from build123d import *

# Parameters (mm, degrees)
F0_W          = 15
F0_H          = 40
F0_W_2        = 20
F0_H_2        = 15
F1_DEPTH      = 30
F2_R          = 25
F2_R_2        = 15
F3_DEPTH      = 20
F3_DEPTH_BACK = 20
F4_DEPTH      = 60
F4_DEPTH_BACK = 60
F5_R          = 12
F7_DEPTH      = 30


with BuildPart() as f1:
    # F0 (on Top) → F1 (new body)
    with BuildSketch(Plane.XY):
        with Locations((-42.5, 20)):
            Rectangle(F0_W, F0_H)
        with BuildLine():
            ThreePointArc((-35, 40), (-29.638939348, 56.069469674), (-20, 70))
            Line((-20, 70), (-20, 85))
            ThreePointArc((-20, 85), (-39.1974084264, 65.2982722843), (-50, 40))
            Line((-50, 40), (-35, 40))
        make_face()
        with Locations((-10, 77.5)):
            Rectangle(F0_W_2, F0_H_2)
        with Locations((10, 77.5)):
            Rectangle(F0_W_2, F0_H_2)
        with BuildLine():
            ThreePointArc((20, 70), (29.638939348, 56.069469674), (35, 40))
            Line((35, 40), (50, 40))
            ThreePointArc((50, 40), (39.1974084264, 65.2982722843), (20, 85))
            Line((20, 85), (20, 70))
        make_face()
        with Locations((42.5, 20)):
            Rectangle(F0_W, F0_H)
    extrude(amount=F1_DEPTH)



with BuildPart() as f3:
    # F2 (on Right) → F3 (new body, two sides)
    with BuildSketch(Plane.YZ) as f3_sk:
        with Locations((0, 15)):
            Circle(F2_R)
        with Locations((0, 15)):
            Circle(F2_R_2, mode=Mode.SUBTRACT)
    extrude(amount=F3_DEPTH)
    extrude(f3_sk.sketch, amount=-F3_DEPTH_BACK)


with BuildPart() as f4:
    # F2 (on Right) → F4 (new body, two sides)
    with BuildSketch(Plane.YZ) as f4_sk:
        with Locations((0, 15)):
            Circle(F2_R_2)
    extrude(amount=F4_DEPTH)
    extrude(f4_sk.sketch, amount=-F4_DEPTH_BACK)

    # F5
    f5_edges = [f4.edges().sort_by_distance(p)[0] for p in [
        (-60, -15, 15),
        (60, -15, 15),
    ]]
    fillet(f5_edges, radius=F5_R)


with BuildPart() as f1_1:
    add(f1.part)

    add(f3.part)  # F7 merges F3

    add(f4.part)  # F7 merges F4
    # F6 (on face) → F7 (join)
    with BuildSketch(Plane(origin=(-50, 0, 0), x_dir=(0, -1, 0), z_dir=(-1, 0, 0))):
        with BuildLine():
            ThreePointArc((0, 0), (-15, 15), (0, 30))
            Line((0, 30), (-5.5677643628, 30))
            ThreePointArc((-5.5677643628, 30), (-16, 15), (-5.5677643628, 0))
            Line((-5.5677643628, 0), (0, 0))
        make_face()
        with BuildLine():
            Line((-5.5677643628, 30), (0, 30))
            ThreePointArc((0, 30), (10.6066017178, 25.6066017178), (15, 15))
            ThreePointArc((15, 15), (10.6066017178, 4.3933982822), (0, 0))
            Line((0, 0), (-5.5677643628, 0))
            ThreePointArc((-5.5677643628, 0), (9.1355287257, 1.8644712743), (16, 15))
            ThreePointArc((16, 15), (9.1355287257, 28.1355287257), (-5.5677643628, 30))
        make_face()
    extrude(amount=-F7_DEPTH)

    # F8: F1 across plane


with BuildPart() as f1_2:
    add(f1_1.part)
    add(f1_1.part.mirror(Plane.YZ))


solid = f1_2.part
Design review of the part built by this model. Coordinates are the model's own, in mm. A direction names the side the tool comes from. Round coordinates to 2 decimals unless told otherwise and drop trailing zeros. Loops run counter-clockwise (first coordinate to the right, second up) from the corner with the lowest first, then second, coordinate; pieces in that order, holes last. Notation, with made-up numbers: (5, 25.25) -> (62, 25.25) arc R26 cw to (62, 45.25) -> close; hole circle Ø11 at (3, 49.25). An arc over 180 degrees is marked (long way). Use one line per item in the form item = value. Start each with the question number.
Q1. We need section B-B on x = 8.5. Give the boundary of the cut face in (y, z).
Q2. We need section A-A on y = 66.5. Give the boundary of the cut face in (x, z).
Q3. For pin 1 Ø1.5 at (y, z) = (63, 28) entering from +X; pin 2 Ø8 at (y, z) = (21.5, 16.5) entering from -X; pin 3 Ø24 at (y, z) = (28, 18.5) entering from +X, all flat-tipped, find the tip position at first contact; note any pin that passes through.
Q4. We need section D-D on z = -6. Give the boundary of the cut face in (x, y), then the cut area to 3 significant figures.
Q5. Wall thickness on line 1 along X through (y, z) = (40, 5); line 2 along X through (y, z) = (18, 21); line 3 along Z through (x, y) = (-12, 79): over which ranges is each line inside the solid? List them lowest first. Write a range as [from, to].
Q6. Draft analysis for pull direction X (two halves, no side actions). For faces 4 (the face through (-20, -0.3, -1.3)), 5 (the face through (50, 25, 15)), 6 (the face through (-38.98, 65.62, 14.79)), state which applies: +X half, -X half, draft (parallel to the pull), parting line (faces both ways), or undercut.
Q7. Machinability: for faces 1 (the face through (-29.745, 55.856, 14.79)), 2 (the face through (39.41, 64.98, 14.79)), 3 (the face through (20, -0.3, -1.3)), which of the approach directions +Z, -Z, +X, -X, +Y, -Y give a long, thin tool a straight path to every point of the face, cutting with its end or side? Answer none if there is none.
Q8. We need section C-C on x = -30.5. Give the boundary of the cut face in (y, z).
Calculated:
q1.outline = circle Ø50 at (0, 15); (70, 0) -> (85, 0) -> (85, 30) -> (70, 30) -> close
q2.outline = (-38.38, 0) -> (-23, 0) -> (-23, 30) -> (-38.38, 30) -> close; (23, 0) -> (38.38, 0) -> (38.38, 30) -> (23, 30) -> close
q3.pin_1 = 41.13
q3.pin_2 = -50
q3.pin_3 = 50
q4.outline = (-20, -13.56) -> (20, -13.56) -> (20, 13.56) -> (-20, 13.56) -> close
q4.area = 1,090 mm²
q5.line_1 = [-50, -35], [35, 50]
q5.line_2 = [-50, -35], [-20, 20], [35, 50]
q5.line_3 = [0, 30]
q6.face_4 = undercut
q6.face_5 = +X half
q6.face_6 = -X half
q7.face_1 = +Z, -Z
q7.face_2 = +Z, -Z, +X, +Y
q7.face_3 = none
q8.outline = circle Ø32 at (0, 15); (54.27, 0) -> (76.05, 0) -> (76.05, 30) -> (54.27, 30) -> close
